from build123d import *

# Parameters (mm, degrees)
F0_W          = 165.1
F0_H          = 25.4
F1_DEPTH      = 16.51
F3_R          = 2.8575
F4_DEPTH      = 8.382
F4_DEPTH_BACK = 33.782
F5_DEPTH      = 25.4
F6_DEPTH      = 25.4
F7_R          = 4.064
F8_DEPTH      = 25.4
F9_R          = 2.54
F10_DEPTH     = 25.4
F11_R         = 3.429
F12_DEPTH     = 3.81
F13_R         = 1.524
F14_R         = 0.762


# Not quite as in the source:
# - a feature names something its author has since deleted; it is built from what else it names


with BuildPart() as f1:
    # F0 (on Front) → F1 (new body)
    with BuildSketch(Plane.XZ):
        with Locations((17.2861106694, 1.5442719363)):
            Rectangle(F0_W, F0_H)
    extrude(amount=F1_DEPTH)

    # F3 (on face) → F4 (join, two sides)
    with BuildSketch(Plane(origin=(0, 0, -11.1557280637), x_dir=(1, 0, 0), z_dir=(0, 0, -1))) as f4_sk:
        with Locations((-46.4608334005, 4.2803706601)):
            Circle(F3_R)
    extrude(amount=F4_DEPTH)
    extrude(f4_sk.sketch, amount=-F4_DEPTH_BACK)

    # F2 (on face) → F5 (join)
    with BuildSketch(Plane(origin=(0, 0, -11.1557280637), x_dir=(1, 0, 0), z_dir=(0, 0, -1))):
        Polygon((99.8361106694, 0), (82.7972726808, 0), (99.8361106694, -15.24), align=None)
    extrude(amount=-F5_DEPTH)

    # F2 (on face) → F6 (join)
    with BuildSketch(Plane(origin=(0, 0, -11.1557280637), x_dir=(1, 0, 0), z_dir=(0, 0, -1))):
        Polygon((99.8361106694, 0), (82.7972726808, 0), (99.8361106694, -15.24), align=None)
    extrude(amount=-F6_DEPTH)

    # F7 (on face) → F8 (cut)
    with BuildSketch(Plane(origin=(0, 0, -11.1557280637), x_dir=(1, 0, 0), z_dir=(0, 0, -1))):
        with Locations((58.2425315266, 16.51)):
            Circle(F7_R)
    extrude(amount=-F8_DEPTH, mode=Mode.SUBTRACT)

    # F9 (on face) → F10 (join)
    with BuildSketch(Plane(origin=(-65.2638893306, 0, 0), x_dir=(0, -1, 0), z_dir=(-1, 0, 0))):
        with Locations((8.255, 1.5442719363)):
            Circle(F9_R)
    extrude(amount=F10_DEPTH)

    # F11 (on face) → F12 (join)
    with BuildSketch(Plane(origin=(-90.6638893306, 0, 0), x_dir=(0, -1, 0), z_dir=(-1, 0, 0))):
        with Locations((8.255, 1.5442719363)):
            Circle(F11_R)
    extrude(amount=F12_DEPTH)

    # F13
    f13_edges = [f1.edges().sort_by_distance(p)[0] for p in [
        (-94.473889, -4.826, 1.544272),
    ]]
    fillet(f13_edges, radius=F13_R)

    # F14
    f14_edges = [f1.edges().sort_by_distance(p)[0] for p in [
        (-90.663889, -4.826, 1.544272),
    ]]
    fillet(f14_edges, radius=F14_R)


solid = f1.part
Source: CAD feature listing. Evaluate the final solid. Frame: model axes, mm. A direction names the side the tool comes from. Give positions to 0.01 mm unless a question says otherwise; leave off trailing zeros. Loops run counter-clockwise (first coordinate to the right, second up) from the corner with the lowest first, then second, coordinate; pieces in that order, holes last. Notation, with made-up numbers: (35.5, 82) -> (93.5, 82) arc R31 ccw to (93.5, 107) -> close; hole circle Ø7 at (68, -21). An arc over 180 degrees is marked (long way). Use a Markdown table: item, result. Add a question column.
1) Pull-direction query (X, two-part tool) for faces 1 (the face through (16, -8, 14.244)), 2 (the face through (-77.79, -6.24, 0)), 3 (the face through (-48.728, -2.542, -15.288)), 4 (the face through (99.836, 0, 1)); classes: +X half, -X half, draft (parallel to the pull), parting line (faces both ways), or undercut.
2) Reachability of faces 5 (the face through (-48.728, -2.542, 18.377)), 6 (the face through (-92.177, -11.526, 2.574)), 7 (the face through (8, 0, 2)), 8 (the face through (-94.474, -8, 2)) from +Z, -Z, +X, -X, +Y, -Y: full face, straight path, thin tool, end or side. Return the list, or none.
3) Section query D-D, the plane y = 13.5. Return the cut outline in (x, z).
4) Section query B-B, the plane y = -14.5. Return the cut outline in (x, z).
5) First-contact query: pin 1 (5 mm diameter, centred on y = 3, z = -12, fed in from +X); pin 2 (7.5 mm diameter, centred on x = 32, z = 6, fed in from +Y); pin 3 (3 mm diameter, centred on x = 31, z = 17.5, fed in from -Y); pin 4 (2 mm diameter, centred on x = -10, y = -9, fed in from -Z). Flat tips, straight axial feed; report the tip coordinate or a pass-through.
6) Section query A-A, the plane z = -9. Return the cut outline in (x, y), then the cut area to 3 significant figures.
7) Section query C-C, the plane x = -59.5. Return the cut outline in (y, z).
8) Line query: line 1 along X through (y, z) = (-5, 12.5); line 2 along Y through (x, z) = (-39, 0); line 3 along Z through (x, y) = (50, -13). Output: solid intervals per line, ascending. Write a range as [from, to].
Numbers:
| question | item | result |
|---|---|---|
| 1 | face 1 | draft |
| 1 | face 2 | undercut |
| 1 | face 3 | parting line |
| 1 | face 4 | +X half |
| 2 | face 5 | +Z |
| 2 | face 6 | -X |
| 2 | face 7 | +Z, -Z, -X, +Y |
| 2 | face 8 | +Z, -Z, -X, +Y, -Y |
| 3 | outline | (97.89, -11.16) -> (99.84, -11.16) -> (99.84, 14.24) -> (97.89, 14.24) -> close |
| 4 | outline | (-65.26, -11.16) -> (54.71, -11.16) -> (54.71, 14.24) -> (-65.26, 14.24) -> close; (61.77, -11.16) -> (99.84, -11.16) -> (99.84, 14.24) -> (61.77, 14.24) -> close |
| 5 | pin 1 | stops at x = 99.84 |
| 5 | pin 2 | stops at y = 0 |
| 5 | pin 3 | passes through |
| 5 | pin 4 | stops at z = -11.16 |
| 6 | outline | (-65.26, -16.51) -> (54.18, -16.51) arc R4.06 cw to (62.31, -16.51) -> (99.84, -16.51) -> (99.84, 15.24) -> (82.8, 0) -> (-65.26, 0) -> close |
| 6 | area | 2,830 mm2 |
| 7 | outline | (-16.51, -11.16) -> (0, -11.16) -> (0, 14.24) -> (-16.51, 14.24) -> close |
| 8 | line 1 | x = [-65.26, 99.84] |
| 8 | line 2 | y = [-16.51, 0] |
| 8 | line 3 | z = [-11.16, 14.24] |
